Work out the finished part from the listing and answer in its coordinate system (mm). A direction names the side the tool comes from. Coordinates: 2 decimals unless noted, no trailing zeros. Order: outer loops, then holes, each group sorted by start corner. A loop starts at its lowest first (then second) coordinate and runs counter-clockwise, first axis right, second up. Notation, with made-up numbers: (82.5, -16) -> (122.5, -16) arc R26 ccw to (122.5, 15) -> close; hole circle Ø8 at (58, 53.25). An arc over 180 degrees is marked (long way). Answer as CSV lines item,"result". Start each with the question number.
Item 1: Section C-C (y = -0.4) is taken. Write down the section's boundary in (x, z).
Item 2: Section D-D (x = -0.5) is taken. Write down the section's boundary in (y, z).
Item 3: For a pull along X with two mould halves and no side action, classify faces 1 (the face through (-5, 0, 13)), 2 (the face through (-3.4, -0.5, 20.828)), 3 (the face through (1.27, -1, 13)) as pulls with the +X half, pulls with the -X half, needs draft (parallel to the pull), parting line crosses it, or undercut.
Item 4: Straight lines are drawn through the part: L1, parallel to Z at x = -3, y = -0.55; L2, parallel to X at y = -1, z = 22; L3, parallel to X at y = -1.7, z = 7. For each, find the intervals that lie inside material, in ascending order.
Item 5: Which of the six approach directions +Z, -Z, +X, -X, +Y, -Y give full straight-line access (tool end or side, diameter ignored) to faces 4 (the face through (-11.1, -2.54, 16.9)), 5 (the face through (-3.4, -0.5, 20.32)), 6 (the face through (-5, -1, 25.4)), 7 (the face through (-11.684, -1, 13))?
Item 6: Each of these flat-tipped pins is pushed along its axis until it touches: pin 1 Ø5 at (x, z) = (-4.5, 15) entering from -Y; pin 2 Ø0.5 at (x, y) = (-8, -0.5) entering from +Z; pin 3 Ø0.5 at (y, z) = (-0.5, 19.5) entering from -X. Where does it stop, or does it pass through?
Item 7: Section A-A (z = 18.5) is taken. Count the separate pieces of the cut face and the enclosed holes in it, then the cut area to 3 significant figures.
```python
from build123d import *

# Parameters (mm, degrees)
F1_DEPTH  = 2.54
F0_W      = 0.508
F0_H      = 0.508
F0_H_2    = 2.032
F0_W_2    = 3.175
F0_H_3    = 2.54
F2_DEPTH  = 1.27
F3_DEPTH  = 1.778
F4_R      = 0.50799
F5_R      = 0.25399
F6_W      = 1.27
F6_H      = 25.4
F7_DEPTH  = 1.27
F8_W      = 1.27
F8_H      = 25.4
F9_DEPTH  = 1.27
F11_DEPTH = 1.27
F12_R     = 0.508


# Not quite as in the source:
# - a fillet or chamfer is up to 0.001 mm smaller than in the source, because OpenCascade refuses the exact size


with BuildPart() as f1:
    # F0 (on Front) → F1 (new body)
    with BuildSketch(Plane.XZ):
        Polygon((0, 24.13), (0, 0), (1.27, 0), (1.27, 25.4), (-11.684, 25.4), (-11.684, 0), (-10.414, 0), (-10.414, 24.13), align=None)
    extrude(amount=F1_DEPTH)

    # F0 (on Front) → F2 (join)
    with BuildSketch(Plane.XZ):
        Polygon((-1.778, 0), (0, 0), (0, 24.13), (-10.414, 24.13), (-10.414, 0), align=None)
        with BuildLine():
            ThreePointArc((-1.2223680419, 10.7806390151), (-1.3851088746, 10.3877478897), (-1.778, 10.2250070571))
            ThreePointArc((-1.778, 10.2250070571), (-2.1708911254, 11.1735301405), (-1.2223680419, 10.7806390151))
        make_face(mode=Mode.SUBTRACT)
        Polygon((-4.953, 22.86), (-1.778, 22.86), (-1.778, 20.828), (-1.778, 20.32), (-1.778, 17.78), (-4.953, 17.78), (-5.461, 17.78), (-8.636, 17.78), (-8.636, 20.32), (-8.636, 20.828), (-8.636, 22.86), (-5.461, 22.86), align=None, mode=Mode.SUBTRACT)
        with Locations((-5.207, 20.574)):
            Rectangle(F0_W, F0_H)
        with Locations((-5.207, 21.844)):
            Rectangle(F0_W, F0_H_2)
        with Locations((-7.0485, 20.574)):
            Rectangle(F0_W_2, F0_H)
        with Locations((-5.207, 19.05)):
            Rectangle(F0_W, F0_H_3)
        with Locations((-3.3655, 20.574)):
            Rectangle(F0_W_2, F0_H)
        with BuildLine():
            ThreePointArc((-1.2223680419, 10.7806390151), (-2.1708911254, 11.1735301405), (-1.778, 10.2250070571))
            ThreePointArc((-1.778, 10.2250070571), (-1.3851088746, 10.3877478897), (-1.2223680419, 10.7806390151))
        make_face()
    extrude(amount=F2_DEPTH)

    # F0 (on Front) → F3 (join)
    with BuildSketch(Plane.XZ):
        with BuildLine():
            ThreePointArc((-1.2223680419, 10.7806390151), (-2.1708911254, 11.1735301405), (-1.778, 10.2250070571))
            ThreePointArc((-1.778, 10.2250070571), (-1.3851088746, 10.3877478897), (-1.2223680419, 10.7806390151))
        make_face()
    extrude(amount=F3_DEPTH)

    # F4 (radius 0.508 in the source; OpenCascade refuses exactly that, so slightly less here)
    f4_edges = [f1.edges().sort_by_distance(p)[0] for p in [
        (-10.414, -2.54, 12.065),
        (0, -2.54, 12.065),
        (-5.207, -2.54, 24.13),
        (-1.778, -1.778, 11.336271),
    ]]
    fillet(f4_edges, radius=F4_R)

    # F5 (radius 0.254 in the source; OpenCascade refuses exactly that, so slightly less here)
    f5_edges = [f1.edges().sort_by_distance(p)[0] for p in [
        (-3.3655, -1.27, 22.86),
        (-1.778, -1.27, 21.844),
        (-3.3655, -1.27, 20.828),
        (-1.778, -1.27, 19.05),
        (-3.3655, -1.27, 17.78),
        (-7.0485, -1.27, 17.78),
        (-5.461, -1.27, 19.05),
        (-7.0485, -1.27, 22.86),
        (-8.636, -1.27, 21.844),
        (-8.636, -1.27, 19.05),
        (-7.0485, -1.27, 20.32),
        (-4.953, -1.27, 21.844),
        (-7.0485, -1.27, 20.828),
        (-5.461, -1.27, 21.844),
        (-4.953, -1.27, 19.05),
        (-3.3655, -1.27, 20.32),
    ]]
    fillet(f5_edges, radius=F5_R)

    # F6 (on face) → F7 (join)
    with BuildSketch(Plane.YZ.offset(1.27)):
        with Locations((-1.905, 12.7)):
            Rectangle(F6_W, F6_H)
    extrude(amount=F7_DEPTH)

    # F8 (on face) → F9 (join)
    with BuildSketch(Plane(origin=(-11.684, 0, 0), x_dir=(0, -1, 0), z_dir=(-1, 0, 0))):
        with Locations((1.905, 12.7)):
            Rectangle(F8_W, F8_H)
    extrude(amount=F9_DEPTH)

    # F10 (on face) → F11 (join)
    with BuildSketch(Plane.XY.offset(25.4)):
        Polygon((-12.954, -1.27), (-12.954, -2.54), (2.54, -2.54), (2.54, -1.27), (1.27, -1.27), (-11.684, -1.27), align=None)
    extrude(amount=F11_DEPTH)

    # F12
    f12_edges = [f1.edges().sort_by_distance(p)[0] for p in [
        (-12.954, -2.54, 13.335),
        (-5.207, -2.54, 26.67),
        (2.54, -2.54, 13.335),
    ]]
    fillet(f12_edges, radius=F12_R)


solid = f1.part
```
Checked values:
1,outline,"(-11.68, 0) -> (1.27, 0) -> (1.27, 25.4) -> (-11.68, 25.4) -> close; hole (-8.64, 17.78) -> (-5.46, 17.78) -> (-5.46, 20.32) -> (-8.64, 20.32) -> close; hole (-8.64, 20.83) -> (-5.46, 20.83) -> (-5.46, 22.86) -> (-8.64, 22.86) -> close; hole (-4.95, 17.78) -> (-1.78, 17.78) -> (-1.78, 20.32) -> (-4.95, 20.32) -> close; hole (-4.95, 20.83) -> (-1.78, 20.83) -> (-1.78, 22.86) -> (-4.95, 22.86) -> close"
2,outline,"(-2.54, 24.64) arc R0.51 ccw to (-2.03, 24.13) -> (-1.27, 24.13) -> (-1.27, 0) -> (0, 0) -> (0, 25.4) -> (-1.27, 25.4) -> (-1.27, 26.67) -> (-2.03, 26.67) arc R0.51 ccw to (-2.54, 26.16) -> close"
3,face 1,"needs draft"
3,face 2,"undercut"
3,face 3,"pulls with the +X half"
4,L1,"z = 0 to 17.78, 20.32 to 20.83, 22.86 to 25.4"
4,L2,"x = -11.68 to -8.64, -5.46 to -4.95, -1.78 to 1.27"
4,L3,"x = -12.95 to -10.41, 0 to 2.54"
5,face 4,"+Z, -Z, +X, -X, -Y"
5,face 5,"+Y, -Y"
5,face 6,"+Z, +X, -X, +Y"
5,face 7,"+Z, -Z, -X, +Y"
6,pin 1,"stops at y = -1.27"
6,pin 2,"stops at z = 25.4"
6,pin 3,"stops at x = -11.68"
7,separate pieces,"3"
7,enclosed holes,"0"
7,area,"14.6 mm^2"
